Design review of the part built by this model. Coordinates are the model's own, in mm. A direction names the side the tool comes from. Coordinates: 2 decimals unless noted, no trailing zeros. Loops run counter-clockwise (first coordinate to the right, second up) from the corner with the lowest first, then second, coordinate; pieces in that order, holes last. Notation, with made-up numbers: (40.25, 63) -> (52.25, 63) arc R29 ccw to (52.25, 100) -> close; hole circle Ø3 at (26, 50). An arc over 180 degrees is marked (long way). Answer as a JSON object with one key per item and string values.
```python
from build123d import *

# Parameters (mm, degrees)
F0_R       = 50.8
F1_DEPTH   = 476.25
F3_R       = 28.575
F4_DEPTH   = 41.402
F1_FACE_R  = 50.8
F4_FACE_R  = 28.575
F1_FACE1_R = 50.8
F5_FACE_R  = 28.575


with BuildPart() as f1:
    # F0 (on Right) → F1 (new body, symmetric)
    with BuildSketch(Plane.YZ):
        Circle(F0_R)
    extrude(amount=F1_DEPTH, both=True)



with BuildPart() as f4:
    # F3 (on offset) → F4 (new body)
    with BuildSketch(Plane.YZ.offset(638.302)):
        Circle(F3_R)
    extrude(amount=-F4_DEPTH)


with BuildPart() as f5_1:
    # F5: instance of F4
    add(f4.part.mirror(Plane.YZ))


with BuildPart() as f1_1:
    add(f1.part)

    add(f4.part)  # F6 merges F4
    # F1_face (on face) → F6 section 0
    with BuildSketch(Plane.YZ.offset(476.25)):
        Circle(F1_FACE_R)
    # F4_face (on face) → F6 section 1
    with BuildSketch(Plane(origin=(596.9, 0, 0), x_dir=(0, 1, 0), z_dir=(-1, 0, 0))):
        Circle(F4_FACE_R)
    loft()


    add(f5_1.part)  # F7 merges F5_1
    # F1_face1 (on face) → F7 section 0
    with BuildSketch(Plane(origin=(-476.25, 0, 0), x_dir=(0, 1, 0), z_dir=(-1, 0, 0))):
        Circle(F1_FACE1_R)
    # F5_face (on face) → F7 section 1
    with BuildSketch(Plane.YZ.offset(-596.9)):
        Circle(F5_FACE_R)
    loft()


solid = f1_1.part
```
1) For faces 1 (the cylindrical face through (617.891, -28.547, 1.256)), 2 (the cylindrical face through (6.668, -11.012, -49.592)), 3 (the cylindrical face through (-617.891, -28.547, 1.256)), list the 3-axis set-ups (+Z, -Z, +X, -X, +Y, -Y) from which the entire face can be reached by the end or side of a thin tool; tool diameter is ignored.
Completed:
{"face 1": "+X", "face 2": "+X, -X", "face 3": "-X"}
2) Add section A-A, the plane y = 0. Give the boundary of the cut face in (x, z) (3 decimals), and give its area (3 significant figures).
Completed:
{"outline": "(-638.302, -28.575) -> (-596.9, -28.575) -> (-476.25, -50.8) -> (476.25, -50.8) -> (596.9, -28.575) -> (638.302, -28.575) -> (638.302, 28.575) -> (596.9, 28.575) -> (476.25, 50.8) -> (-476.25, 50.8) -> (-596.9, 28.575) -> (-638.302, 28.575) -> close", "area": "121,000 mm²"}
3) Add section B-B, the plane x = -368. Give the boundary of the cut face in (y, z).
Completed:
{"outline": "circle Ø101.6 at (0, 0)"}
4) Wall thickness on probe 1 along Y at (x, z) = (345, -2); probe 2 along Y at (x, z) = (-133.5, -5): over which ranges is each line inside the solid? List them lowest first.
Completed:
{"probe 1": "-50.76 to 50.76", "probe 2": "-50.55 to 50.55"}
5) Clearance check with flat-ended pins moving along their axes: pin 1 Ø12 at (x, z) = (19.5, 26.5) entering from -Y; pin 2 Ø12 at (x, z) = (33.5, -20) entering from +Y; pin 3 Ø4 at (x, z) = (-320, -13.5) entering from +Y. State where each tip first meets the part, or that it passes through.
Completed:
{"pin 1": "y = -46.48", "pin 2": "y = 48.83", "pin 3": "y = 49.48"}
